from build123d import *

# Parameters (mm, degrees)
SKETCH1_W           = 41
SKETCH1_H           = 38
BOSS_EXTRUDE1_DEPTH = 10
SKETCH2_R           = 10
SKETCH2_R_2         = 5
CUT_EXTRUDE1_DEPTH  = 2
CUT_EXTRUDE2_REACH  = 12
SKETCH2_2_R         = 5
FILLET1_R           = 14
BOSS_EXTRUDE2_DEPTH = 10
BOSS_EXTRUDE3_DEPTH = 2
BOSS_EXTRUDE4_DEPTH = 5


with BuildPart() as part:
    # Sketch1 → Boss-Extrude1 (new body)
    with BuildSketch(Plane(origin=(0, 0, 0), x_dir=(1, 0, 0), z_dir=(0, 1, 0))):
        with Locations((-20.5, -19)):
            Rectangle(SKETCH1_W, SKETCH1_H)
    extrude(amount=BOSS_EXTRUDE1_DEPTH)

    # Sketch2 → Cut-Extrude1 (cut)
    with BuildSketch(Plane(origin=(0, 10, 0), x_dir=(1, 0, 0), z_dir=(0, 1, 0))):
        with Locations((-27, -24)):
            Circle(SKETCH2_R)
        with Locations((-27, -24)):
            Circle(SKETCH2_R_2, mode=Mode.SUBTRACT)
    extrude(amount=-CUT_EXTRUDE1_DEPTH, mode=Mode.SUBTRACT)

    # Sketch2_2 → Cut-Extrude2 (cut, up to next)
    with BuildSketch(Plane(origin=(0, 10, 0), x_dir=(1, 0, 0), z_dir=(0, 1, 0)), mode=Mode.PRIVATE) as cut_extrude2_sk1:
        with Locations((-27, -24)):
            Circle(SKETCH2_2_R)
    cut_extrude2_tool1 = extrude(cut_extrude2_sk1.sketch, amount=-CUT_EXTRUDE2_REACH, mode=Mode.PRIVATE) & part.part
    add(cut_extrude2_tool1.solids().sort_by_distance((-27, 10, 24))[0], mode=Mode.SUBTRACT)

    # Fillet1
    fillet1_edges = [part.edges().sort_by_distance(p)[0] for p in [
        (-41, 5, 38),
    ]]
    fillet(fillet1_edges, radius=FILLET1_R)

    # Sketch4 → Boss-Extrude2 (add)
    with BuildSketch(Plane.XY):
        with BuildLine():
            ThreePointArc((0, 77), (-10.488696893, 73.842576731), (-17.491366878, 65.419709208))
            Line((-17.491366878, 65.419709208), (-41, 10))
            Line((-41, 10), (0, 10))
            Line((0, 10), (0, 47))
            ThreePointArc((0, 47), (-11, 58), (0, 69))
            Line((0, 69), (0, 77))
        make_face()
    extrude(amount=BOSS_EXTRUDE2_DEPTH)

    # Sketch5 → Boss-Extrude3 (add)
    with BuildSketch(Plane(origin=(0, 0, 0), x_dir=(-1, 0, 0), z_dir=(0, 0, -1))):
        with BuildLine():
            Line((0, 47), (0, 39))
            ThreePointArc((0, 39), (13.435028843, 44.564971157), (19, 58))
            ThreePointArc((19, 58), (18.619022137, 61.785764739), (17.491366878, 65.419709208))
            ThreePointArc((17.491366878, 65.419709208), (10.488696893, 73.842576731), (0, 77))
            Line((0, 77), (0, 69))
            ThreePointArc((0, 69), (11, 58), (0, 47))
        make_face()
    extrude(amount=BOSS_EXTRUDE3_DEPTH)

    # Sketch6 → Boss-Extrude4 (add)
    with BuildSketch(Plane(origin=(0, 0, 0), x_dir=(0, 0, -1), z_dir=(1, 0, 0))):
        Polygon((-38, 10), (-10, 40), (-10, 10), align=None)
    extrude(amount=-BOSS_EXTRUDE4_DEPTH)

    # Mirror1: part across plane


with BuildPart() as part_1:
    add(part.part)
    add(part.part.mirror(Plane(origin=(0, 10, 0), x_dir=(0, 0, 1), z_dir=(-1, 0, 0))))


solid = part_1.part
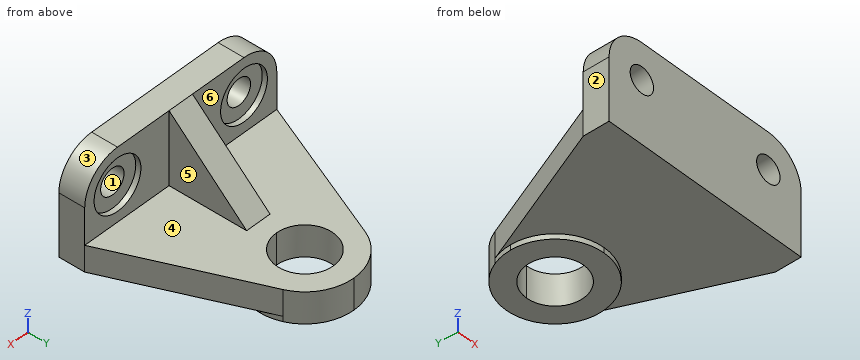
For this review, take the finished solid that the model builds, in its own axes (mm). Face numbers are marked on the shaded views. A direction names the side the tool comes from. Round coordinates to 2 decimals unless told otherwise and drop trailing zeros. Write each loop counter-clockwise with the first axis right and the second up, starting at its lowest first coordinate (ties: lowest second). Pieces come first, ordered by that corner, then holes. Notation, with made-up numbers: (46, 68.25) -> (78, 68.25) arc R17 ccw to (78, 73.25) -> close; hole circle Ø6 at (50.5, 37.5). An arc over 180 degrees is marked (long way). Put each result on its own line as item: value.
Q1. Consider section C-C on x = 35. State the section outline as (y, z) points, and give its area (3 significant figures).
Determined:
outline: (0, 0) -> (24.14, 0) -> (24.14, 10) -> (10, 10) -> (10, 18) -> (8, 18) -> (8, 30) -> (10, 30) -> (10, 35.49) -> (0, 35.49) -> close
area: 472 mm^2
Q2. Consider section B-B on x = 24. State the section outline as (y, z) points.
Determined:
outline: (0, 0) -> (50.08, 0) -> (50.08, 10) -> (10, 10) -> (10, 14.46) -> (8, 14.46) -> (8, 20) -> (0, 20) -> close; (0, 28) -> (8, 28) -> (8, 33.54) -> (10, 33.54) -> (10, 38) -> (0, 38) -> close
Q3. The part is to be moulded in two halves that separate along Z. For the marked faces 1, 2 and 3, say which applies: released by +Z, released by -Z, zero draft, split by the parting line, or undercut.
Determined:
face 1: undercut
face 2: zero draft
face 3: released by +Z
Q4. Clearance check with flat-ended pins moving along their axes: pin 1 Ø16 at (x, z) = (-28.5, 24.5) entering from +Y; pin 2 Ø12 at (y, z) = (52, 17) entering from +X; pin 3 Ø6 at (x, y) = (16.5, 33.5) entering from -Z; pin 4 Ø8.5 at (y, z) = (31.5, 21.5) entering from -X. State where each tip first meets the part, or that it passes through.
Determined:
pin 1: stops at y = 8
pin 2: passes through
pin 3: stops at z = 0
pin 4: stops at x = -5
Q5. To check wall thickness, follow L1, parallel to X at y = 2.5, z = 24; L2, parallel to X at y = 8.55, z = 24; L3, parallel to Z at x = -27, y = 9.5. State the ranges of each line that lie inside material, in increasing order. Write a range as [from, to].
Determined:
L1: x = [-41, -32], [-22, 22], [32, 41]
L2: x = [-41, -37], [-17, 17], [37, 41]
L3: z = [0, 14], [34, 38]
Q6. Consider section D-D on y = 17. State the section outline as (x, z) points.
Determined:
outline: (-38.03, 0) -> (38.03, 0) -> (38.03, 10) -> (5, 10) -> (5, 31.47) -> (-5, 31.47) -> (-5, 10) -> (-38.03, 10) -> close
Q7. Consider section A-A on y = 49.5. State the section outline as (x, z) points.
Determined:
outline: (-24.24, 0) -> (-16.99, 0) -> (-16.99, -2) -> (-6.98, -2) -> (-6.98, 10) -> (-24.24, 10) -> close; (6.98, -2) -> (16.99, -2) -> (16.99, 0) -> (24.24, 0) -> (24.24, 10) -> (6.98, 10) -> close
Q8. Machinability: for the marked faces 4, 5 and 6, which of the approach directions +Z, -Z, +X, -X, +Y, -Y give a long, thin tool a straight path to every point of the face, cutting with its end or side? Answer none if there is none.
Determined:
face 4: +Z, +Y
face 5: +Z, +X, +Y
face 6: +Z, -X, +Y
